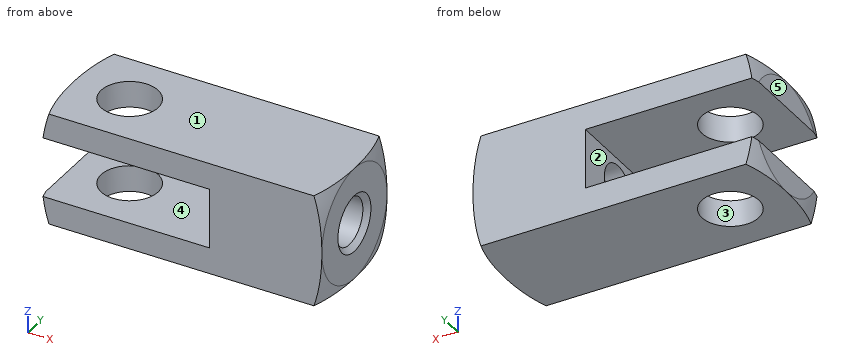
Autodesk Inventor part; units mm, degrees
ref_plane "dummy_XY" through (0, 0, 0) normal (0, 0, 1) x (1, 0, 0)
ref_plane "dummy_YZ" through (0, 0, 0) normal (1, 0, 0) x (0, 1, 0)
ref_plane "dummy_ZX" through (0, 0, 0) normal (0, 1, 0) x (0, 0, 1)
sketch "Sketch_1" plane through (0, 0, 0) normal (0, 0, 1) x (1, 0, 0)
  line L0 (-4.7498, 4.7625) -> (-4.7498, -4.7625)
  line L1 (-4.7498, -4.7625) -> (19.05, -4.7625)
  line L2 (19.05, -4.7625) -> (19.05, 4.7625)
  line L3 (19.05, 4.7625) -> (-4.7498, 4.7625)
extrude "Extrusion1" add sketch "Sketch_1" along normal mid plane 9.525
sketch "Sketch_2" plane through (0, 0, 0) normal (0, 1, 0) x (-1, 0, 0)
  line L0 (4.7498, -2.54) -> (4.7498, 2.54)
  line L1 (4.7498, 2.54) -> (-9.525, 2.54)
  line L2 (-9.525, 2.54) -> (-9.525, -2.54)
  line L3 (-9.525, -2.54) -> (4.7498, -2.54)
extrude "Extrusion2" cut sketch "Sketch_2" along normal mid plane 9.525
sketch "Sketch3" plane through (19.05, -4.7625, 4.7625) normal (1, 0, 0) x (0, 0, -1)
  point P0 (4.7625, 4.7625)
hole "Hole1" at (19.05, 0, 0) direction (-1, 0, 0) diameter 3.9624 depth 7.874 countersink diameter 4.826 countersink angle 90
sketch "Sketch4" plane through (11.176, 0, 0) normal (1, 0, 0) x (0, 0, -1)
  point P0 (0, 0)
hole "Hole2" at (11.176, 0, 0) direction (-1, 0, 0) diameter 3.9675 depth 1.651
sketch "Sketch5" plane through (0, 0, -4.7625) normal (0, 0, -1) x (-1, 0, 0)
  point P0 (0, 0)
hole "Hole3" at (0, 0, -4.7625) direction (0, 0, 1) diameter 4.826 depth 9.525
sketch "Sketch_9" plane through (0, 0, 0) normal (0, 0, 1) x (1, 0, 0)
  line L0 (23.8125, 0) -> (19.05, 0)
  line L1 (19.05, 0) -> (19.05, 4.7625)
  arc A0 (19.05, 4.7625) -> (16.51, 9.525) centre (8.8503, 2.3812) ccw
  line L2 (16.51, 9.525) -> (23.8125, 9.525)
  line L3 (23.8125, 9.525) -> (23.8125, 0)
  line L4 (23.8125, 0) -> (19.05, 0)
revolve "Revolution1" cut sketch "Sketch_9" angle 360 about axis through (23.8125, 0, 0) along (1, 0, 0)
sketch "Sketch_10" plane through (0, 0, 0) normal (0, 0, 1) x (1, 0, 0)
  line L0 (-4.7498, 0) -> (-9.5123, 0)
  line L1 (-9.5123, 0) -> (-9.5123, 9.525)
  line L2 (-9.5123, 9.525) -> (-2.2098, 9.525)
  arc A0 (-2.2098, 9.525) -> (-4.7498, 4.7625) centre (5.4499, 2.3812) ccw
  line L3 (-4.7498, 4.7625) -> (-4.7498, 0)
  line L4 (-4.7498, 0) -> (-9.5123, 0)
revolve "Revolution2" cut sketch "Sketch_10" angle 360 about axis through (-4.7498, 0, 0) along (1, 0, 0)
ref_plane "dummy_XY" through (0, 0, 0) normal (0, 0, 1) x (1, 0, 0)
ref_plane "dummy_YZ" through (0, 0, 0) normal (1, 0, 0) x (0, 1, 0)
ref_plane "dummy_ZX" through (0, 0, 0) normal (0, 1, 0) x (0, 0, 1)
ref_plane "h1_XY" through (-4.7498, 4.7625, 0) normal (0, 0, 1) x (1, 0, 0)
ref_plane "h1_YZ" through (-4.7498, 4.7625, 0) normal (1, 0, 0) x (0, 1, 0)
ref_plane "h1_ZX" through (-4.7498, 4.7625, 0) normal (0, 1, 0) x (0, 0, 1)
ref_plane "h2_XY" through (-4.7498, -4.7625, 0) normal (0, 0, 1) x (1, 0, 0)
ref_plane "h2_YZ" through (-4.7498, -4.7625, 0) normal (1, 0, 0) x (0, 1, 0)
ref_plane "h2_ZX" through (-4.7498, -4.7625, 0) normal (0, 1, 0) x (0, 0, 1)
ref_plane "l1_XY" through (19.05, 4.7625, 0) normal (0, 0, 1) x (1, 0, 0)
ref_plane "l1_YZ" through (19.05, 4.7625, 0) normal (1, 0, 0) x (0, 1, 0)
ref_plane "l1_ZX" through (19.05, 4.7625, 0) normal (0, 1, 0) x (0, 0, 1)
ref_plane "l11_XY" through (19.05, 4.7625, 0) normal (0, 0, 1) x (1, 0, 0)
ref_plane "l11_YZ" through (19.05, 4.7625, 0) normal (1, 0, 0) x (0, 1, 0)
ref_plane "l11_ZX" through (19.05, 4.7625, 0) normal (0, 1, 0) x (0, 0, 1)
ref_plane "l12_XY" through (0, 4.7625, 0) normal (0, 0, 1) x (1, 0, 0)
ref_plane "l12_YZ" through (0, 4.7625, 0) normal (1, 0, 0) x (0, 1, 0)
ref_plane "l12_ZX" through (0, 4.7625, 0) normal (0, 1, 0) x (0, 0, 1)
ref_plane "l2_XY" through (-4.7498, 4.7625, 0) normal (0, 0, 1) x (1, 0, 0)
ref_plane "l2_YZ" through (-4.7498, 4.7625, 0) normal (1, 0, 0) x (0, 1, 0)
ref_plane "l2_ZX" through (-4.7498, 4.7625, 0) normal (0, 1, 0) x (0, 0, 1)
ref_plane "l21_XY" through (19.05, 0, 0) normal (0, 1, 0) x (1, 0, 0)
ref_plane "l21_YZ" through (19.05, 0, 0) normal (1, 0, 0) x (0, 0, -1)
ref_plane "l21_ZX" through (19.05, 0, 0) normal (0, 0, -1) x (0, 1, 0)
ref_plane "l22_XY" through (9.525, 0, 0) normal (0, 1, 0) x (1, 0, 0)
ref_plane "l22_YZ" through (9.525, 0, 0) normal (1, 0, 0) x (0, 0, -1)
ref_plane "l22_ZX" through (9.525, 0, 0) normal (0, 0, -1) x (0, 1, 0)
ref_plane "piston_rod_clevis_XY" through (19.05, 0, 0) normal (1, 0, 0) x (0, 0, -1)
ref_plane "piston_rod_clevis_YZ" through (19.05, 0, 0) normal (0, 0, -1) x (0, 1, 0)
ref_plane "piston_rod_clevis_ZX" through (19.05, 0, 0) normal (0, 1, 0) x (1, 0, 0)
ref_plane "rod_clevis_body_XY" through (0, 0, 0) normal (0, 0, 1) x (1, 0, 0)
ref_plane "rod_clevis_body_YZ" through (0, 0, 0) normal (1, 0, 0) x (0, 1, 0)
ref_plane "rod_clevis_body_ZX" through (0, 0, 0) normal (0, 1, 0) x (0, 0, 1)
ref_plane "th1_XY" through (19.05, 2.413, 0) normal (0, 0, 1) x (1, 0, 0)
ref_plane "th1_YZ" through (19.05, 2.413, 0) normal (1, 0, 0) x (0, 1, 0)
ref_plane "th1_ZX" through (19.05, 2.413, 0) normal (0, 1, 0) x (0, 0, 1)
ref_plane "th2_XY" through (19.05, -2.413, 0) normal (0, 0, 1) x (1, 0, 0)
ref_plane "th2_YZ" through (19.05, -2.413, 0) normal (1, 0, 0) x (0, 1, 0)
ref_plane "th2_ZX" through (19.05, -2.413, 0) normal (0, 1, 0) x (0, 0, 1)
ref_plane "to_cylinder_XY" through (9.525, 0, 0) normal (1, 0, 0) x (0, 0, -1)
ref_plane "to_cylinder_YZ" through (9.525, 0, 0) normal (0, 0, -1) x (0, 1, 0)
ref_plane "to_cylinder_ZX" through (9.525, 0, 0) normal (0, 1, 0) x (1, 0, 0)
ref_plane "w1_XY" through (19.05, 0, -4.7625) normal (0, 1, 0) x (1, 0, 0)
ref_plane "w1_YZ" through (19.05, 0, -4.7625) normal (1, 0, 0) x (0, 0, -1)
ref_plane "w1_ZX" through (19.05, 0, -4.7625) normal (0, 0, -1) x (0, 1, 0)
ref_plane "w11_XY" through (-4.7498, 0, -2.54) normal (0, 1, 0) x (1, 0, 0)
ref_plane "w11_YZ" through (-4.7498, 0, -2.54) normal (1, 0, 0) x (0, 0, -1)
ref_plane "w11_ZX" through (-4.7498, 0, -2.54) normal (0, 0, -1) x (0, 1, 0)
ref_plane "w12_XY" through (-4.7498, 0, 2.54) normal (0, 1, 0) x (1, 0, 0)
ref_plane "w12_YZ" through (-4.7498, 0, 2.54) normal (1, 0, 0) x (0, 0, -1)
ref_plane "w12_ZX" through (-4.7498, 0, 2.54) normal (0, 0, -1) x (0, 1, 0)
ref_plane "w2_XY" through (19.05, 0, 4.7625) normal (0, 1, 0) x (1, 0, 0)
ref_plane "w2_YZ" through (19.05, 0, 4.7625) normal (1, 0, 0) x (0, 0, -1)
ref_plane "w2_ZX" through (19.05, 0, 4.7625) normal (0, 0, -1) x (0, 1, 0)
properties part number "D-14043"
Can you work these out from the model? Positions are in its coordinate system, mm. Face numbers are marked on the shaded views. A direction names the side the tool comes from. Coordinates: 2 decimals unless noted, no trailing zeros. Write each loop counter-clockwise with the first axis right and the second up, starting at its lowest first coordinate (ties: lowest second). Pieces come first, ordered by that corner, then holes. Notation, with made-up numbers: (49.25, -13) -> (104.25, -13) arc R23 cw to (104.25, -1) -> close; hole circle Ø10 at (-0.75, 24.25). An arc over 180 degrees is marked (long way). Answer as CSV lines item,"result".
1) On a 3-axis mill with a long thin cutter (end or side, diameter ignored), from which of +Z, -Z, +X, -X, +Y, -Y can I reach the whole of each face in a straight line? I mean the marked faces 4 and 5. Say none if no direction works.
Check result:
face 4,"-X, +Y, -Y"
face 5,"+Z, -Z, -X, +Y, -Y"
2) If we section it at C-C on x = 10: Please give me the cut outline in (y, z).
Check result:
outline,"(-4.76, -4.76) -> (4.76, -4.76) -> (4.76, 4.76) -> (-4.76, 4.76) -> close; hole circle Ø3.97 at (0, 0)"
3) If I drill on line 1 (Z direction, x = 5.75, y = -4); line 2 (Z direction, x = 13.25, y = 0); line 3 (X direction, y = 0, z = 3.8), over which ranges is the centre line in solid material (lowest first)? Write a range as from..to.
Check result:
line 1,"-4.76..-2.54, 2.54..4.76"
line 2,"-4.76..-1.98, 1.98..4.76"
line 3,"-4.75..-2.41, 2.41..19.05"
4) If we section it at D-D on y = -0.5: Count the separate pieces of the cut face and the enclosed holes in it, then the cut area to 3 significant figures.
Check result:
separate pieces,"4"
enclosed holes,"0"
area,"96.5 mm²"
5) If we section it at B-B on x = 0: Please give me the cut outline in (y, z), then the cut area to 3 significant figures.
Check result:
outline,"(-4.76, -4.76) -> (-2.41, -4.76) -> (-2.41, -2.54) -> (-4.76, -2.54) -> close; (-4.76, 2.54) -> (-2.41, 2.54) -> (-2.41, 4.76) -> (-4.76, 4.76) -> close; (2.41, -4.76) -> (4.76, -4.76) -> (4.76, -2.54) -> (2.41, -2.54) -> close; (2.41, 2.54) -> (4.76, 2.54) -> (4.76, 4.76) -> (2.41, 4.76) -> close"
area,"20.9 mm²"
6) If we mould it in two halves opening along X, with no side actions, what happens to the marked faces 1, 2 and 3? For each: +X half, -X half, draft (parallel to the pull), parting line (faces both ways), or undercut.
Check result:
face 1,"draft"
face 2,"-X half"
face 3,"undercut"
7) If we section it at A-A on x = 6.5: Please give me the cut outline in (y, z).
Check result:
outline,"(-4.76, -4.76) -> (4.76, -4.76) -> (4.76, -2.54) -> (-4.76, -2.54) -> close; (-4.76, 2.54) -> (4.76, 2.54) -> (4.76, 4.76) -> (-4.76, 4.76) -> close"
8) Will this pin go through, and if not, where does the flat tip stop? P1, Ø5, axis at y = 0, z = 0, coming from the -X side (3 decimals).
Check result:
P1,"x = 9.525"
